from build123d import *

# Parameters (mm, degrees)
SKETCH1_W               = 40
SKETCH1_H               = 40
BOSS_EXTRUDE1_DEPTH     = 10
SKETCH2_R               = 2.5
CUT_EXTRUDE1_DEPTH      = 11
MIRROR2_COPY_1_SKETCH_R = 2.5
MIRROR2_COPY_1_DEPTH    = 11
FILLET2_R               = 5


with BuildPart() as part:
    # Sketch1 → Boss-Extrude1 (new body)
    with BuildSketch(Plane.XY):
        with Locations((20, 20)):
            Rectangle(SKETCH1_W, SKETCH1_H)
    extrude(amount=BOSS_EXTRUDE1_DEPTH)

    # Sketch2 → Cut-Extrude1 (cut, through all)
    with BuildSketch(Plane.XY.offset(10)):
        with Locations((5, 35)):
            Circle(SKETCH2_R)
    cut_extrude1 = extrude(amount=-CUT_EXTRUDE1_DEPTH, mode=Mode.SUBTRACT)

    # Mirror1: Cut-Extrude1 across plane
    add(cut_extrude1.mirror(Plane.ZX.offset(20)), mode=Mode.SUBTRACT)

    # Mirror2: Cut-Extrude1 across plane
    add(cut_extrude1.mirror(Plane(origin=(20, 0, 0), x_dir=(0, 0, 1), z_dir=(1, 0, 0))), mode=Mode.SUBTRACT)

    # Mirror2 copy 1 sketch → Mirror2 copy 1 (cut, through all)
    with BuildSketch(Plane(origin=(40, 40, 10), x_dir=(-1, 0, 0), z_dir=(0, 0, 1))):
        with Locations((5, 35)):
            Circle(MIRROR2_COPY_1_SKETCH_R)
    extrude(amount=-MIRROR2_COPY_1_DEPTH, mode=Mode.SUBTRACT)

    # Fillet2
    fillet2_edges = [part.edges().sort_by_distance(p)[0] for p in [
        (0, 40, 5),
        (40, 40, 5),
        (40, 0, 5),
        (0, 0, 5),
    ]]
    fillet(fillet2_edges, radius=FILLET2_R)


solid = part.part
Read the model definition and answer for the solid it produces. Units are mm, in the model's axes. Coordinates: 2 decimals unless noted, no trailing zeros. Write each loop counter-clockwise with the first axis right and the second up, starting at its lowest first coordinate (ties: lowest second). Pieces come first, ordered by that corner, then holes. Notation, with made-up numbers: (-25.75, -17) - (33.25, -17) arc R23 cw to (33.25, -3) - close; hole circle Ø1 at (-38.5, 28). An arc over 180 degrees is marked (long way). One line per question, with ' | ' between items.
Q1. Determine the mould class of faces 1 (the cylindrical face through (7.385, 35.751, 5.07)), 2 (the flat face through (20, 20, 0)), 3 (the flat face through (20, 0, 5)), 4 (the flat face through (20, 40, 5)) for opening direction Y: +Y half, -Y half, draft (parallel to the pull), parting line (faces both ways), or undercut.
Result set:
face 1: undercut | face 2: draft | face 3: -Y half | face 4: +Y half
Q2. Find section B-B, the plane x = 34.5. Write down the section's boundary in (y, z).
Result set:
outline: (0, 0) - (2.55, 0) - (2.55, 10) - (0, 10) - close; (7.45, 0) - (32.55, 0) - (32.55, 10) - (7.45, 10) - close; (37.45, 0) - (40, 0) - (40, 10) - (37.45, 10) - close
Q3. This flat-tipped pin is pushed along its axis until it touches: P1, Ø4.5, axis at x = 5, y = 35, coming from the -Z side. Where does it stop, or does it pass through?
Result set:
P1: through
Q4. Consider L1, parallel to X at y = 5, z = 7.5; L2, parallel to X at y = 36.5, z = 2.25. Determine where each line is inside the solid, lowest interval first. Write a range as [from, to].
Result set:
L1: [0, 2.5], [7.5, 32.5], [37.5, 40] | L2: [0.23, 3], [7, 33], [37, 39.77]
Q5. Find section A-A, the plane z = 4.25. Write down the section's boundary in (x, y).
Result set:
outline: (0, 5) arc R5 ccw to (5, 0) - (35, 0) arc R5 ccw to (40, 5) - (40, 35) arc R5 ccw to (35, 40) - (5, 40) arc R5 ccw to (0, 35) - close; hole circle Ø5 at (5, 5); hole circle Ø5 at (5, 35); hole circle Ø5 at (35, 5); hole circle Ø5 at (35, 35)
